The listing builds one solid part. Answer for the finished solid, in the listing's coordinates (mm). A direction names the side the tool comes from. Round coordinates to 2 decimals unless told otherwise and drop trailing zeros. Write each loop counter-clockwise with the first axis right and the second up, starting at its lowest first coordinate (ties: lowest second). Pieces come first, ordered by that corner, then holes.
from build123d import *

# Parameters (mm, degrees)
F1_DEPTH       = 101.6
F3_D           = 6.35
F3_CBORE_D     = 9.3345
F3_CBORE_DEPTH = 24.4602
F4_W           = 12.7
F4_H           = 63.5
F5_DEPTH       = 22.86
F7_D           = 6.35
F8_R           = 5.08
F9_W           = 16.6624
F9_H           = 10.16
F10_DEPTH      = 19.177


with BuildPart() as f1:
    # F0 (on Front) → F1 (new body)
    with BuildSketch(Plane.XZ):
        with BuildLine():
            Line((0, 38.1), (0, 0))
            Line((0, 0), (88.9, 0))
            Line((88.9, 0), (88.9, 38.1))
            Line((88.9, 38.1), (63.5, 38.1))
            ThreePointArc((63.5, 38.1), (43.307, 17.907), (23.114, 38.1))
            Line((23.114, 38.1), (0, 38.1))
        make_face()
    extrude(amount=-F1_DEPTH)

    # F3 (through all)
    with Locations(Plane.XY.offset(38.1)):
        with Locations((16.5989, 8.1661), (16.5989, 93.4339), (80.0989, 93.4339), (80.0989, 8.1661)):
            CounterBoreHole(F3_D / 2, F3_CBORE_D / 2, F3_CBORE_DEPTH)

    # F4 (on face) → F5 (join)
    with BuildSketch(Plane.XY.offset(38.1)):
        with Locations((82.55, 51.435)):
            Rectangle(F4_W, F4_H)
    extrude(amount=F5_DEPTH)

    # F7 (through all)
    with Locations(Plane.XZ.offset(-19.685)):
        with Locations((82.55, 51.435)):
            Hole(F7_D / 2)

    # F8
    f8_edges = [f1.edges().sort_by_distance(p)[0] for p in [
        (76.2, 51.435, 60.96),
        (88.9, 51.435, 60.96),
    ]]
    fillet(f8_edges, radius=F8_R)

    # F9 (on face) → F10 (cut)
    with BuildSketch(Plane.XY.offset(38.1)):
        with Locations((11.2522, 51.689)):
            Rectangle(F9_W, F9_H)
    extrude(amount=-F10_DEPTH, mode=Mode.SUBTRACT)


solid = f1.part
1. Section A-A on z = 29.5 is taken. Determine the outline of the cut face in (x, y).
Geometry says:
outline: (0, 0) - (25.04, 0) - (25.04, 101.6) - (0, 101.6) - close; (61.58, 0) - (88.9, 0) - (88.9, 101.6) - (61.58, 101.6) - close; hole (2.92, 46.61) - (19.58, 46.61) - (19.58, 56.77) - (2.92, 56.77) - close; hole circle Ø9.33 at (16.6, 8.17); hole circle Ø9.33 at (16.6, 93.43); hole circle Ø9.33 at (80.1, 8.17); hole circle Ø9.33 at (80.1, 93.43)
2. Section C-C on y = 15 is taken. Determine the outline of the cut face in (x, z), plus the area to 3 significant figures.
Geometry says:
outline: (0, 0) - (88.9, 0) - (88.9, 38.1) - (63.5, 38.1) arc R20.19 cw to (23.11, 38.1) - (0, 38.1) - close
area: 2,750 mm2
3. Section D-D on z = 45 is taken. Determine the outline of the cut face in (x, y) (3 decimals), plus the area to 3 significant figures.
Geometry says:
outline: (76.2, 19.685) - (88.9, 19.685) - (88.9, 83.185) - (76.2, 83.185) - close
area: 806 mm2
4. Given pin 1 (3 mm diameter, centred on x = 81, y = 6, fed in from +Z); pin 2 (8 mm diameter, centred on x = 39, y = 70.5, fed in from +Z); pin 3 (4.5 mm diameter, centred on x = 18.5, y = 6.5, fed in from +Z), each flat-ended and moving along its own axis, determine where each tip first touches the part or whether it passes through.
Geometry says:
pin 1: stops at z = 13.64
pin 2: stops at z = 19.69
pin 3: stops at z = 38.1
5. Section B-B on y = 77 is taken. Determine the outline of the cut face in (x, z) (3 decimals).
Geometry says:
outline: (0, 0) - (88.9, 0) - (88.9, 55.88) arc R5.08 ccw to (83.82, 60.96) - (81.28, 60.96) arc R5.08 ccw to (76.2, 55.88) - (76.2, 38.1) - (63.5, 38.1) arc R20.193 cw to (23.114, 38.1) - (0, 38.1) - close; hole circle Ø6.35 at (82.55, 51.435)
6. For a pull along Y with two mould halves and no side action, classify faces 1 (the face through (11, 56.769, 29)), 2 (the face through (44, 101.6, 15)), 3 (the face through (83.238, 51.88, 48.336)) as released by +Y, released by -Y, zero draft, split by the parting line, or undercut.
Geometry says:
face 1: undercut
face 2: released by +Y
face 3: zero draft
7. Straight lines are drawn through the part: line 1 along X through (y, z) = (91, 15); line 2 along Z through (x, y) = (84, 17.5); line 3 along Y through (x, z) = (78.5, 33). For each, find the intervals that lie inside material, in ascending order.
Geometry says:
line 1: x = 0 to 12.62, 20.58 to 76.12, 84.08 to 88.9
line 2: z = 0 to 38.1
line 3: y = 0 to 3.78, 12.55 to 89.05, 97.82 to 101.6
8. A tool of negligible diameter and unlimited length cuts with its end or side. For faces 4 (the face through (84.55, 9.57, 26.04)), 5 (the face through (88.9, 50, 21)), 6 (the face through (1, 50, 38.1)), from which of +Z, -Z, +X, -X, +Y, -Y can it reach the whole face along a straight path? Write none if from no direction.
Geometry says:
face 4: +Z
face 5: +Z, -Z, +X, +Y, -Y
face 6: +Z, -X, +Y, -Y
